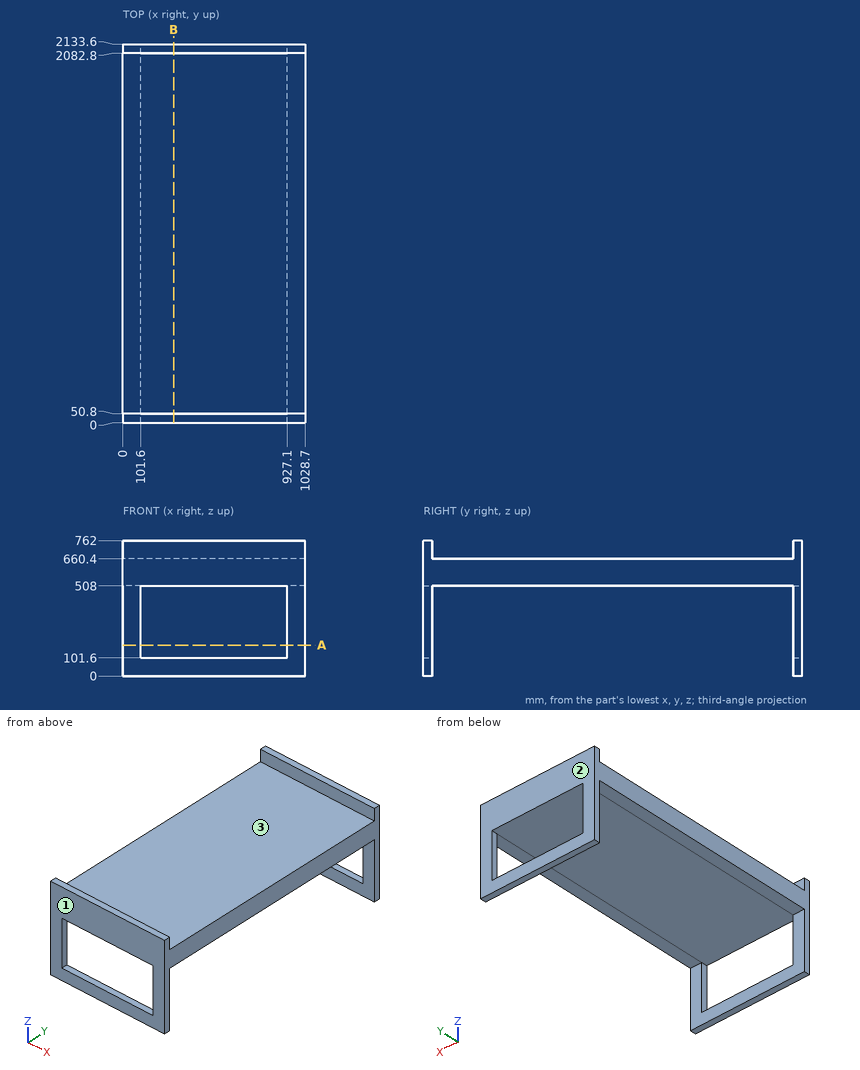
Could you check a few things on this drawing? It's one solid part, dimensions in mm from its lowest x, y, z. Coordinates: 2 decimals unless noted, no trailing zeros. Loops run counter-clockwise (first coordinate to the right, second up) from the corner with the lowest first, then second, coordinate; pieces in that order, holes last. Notation, with made-up numbers: (51, 35) - (81, 35) arc R22 ccw to (81, 59) - close; hole circle Ø11 at (34, -38). An arc over 180 degrees is marked (long way). Answer as a JSON object with one key per item and string values. Group by question number.
Item 1: If we section it at A-A (z = 174): List the corners of the cut face in (x, y) for me, plus the area to 3 significant figures.
Item 2: If we section it at B-B (x = 286): List the corners of the cut face in (y, z) for me, plus the area to 3 significant figures.
Item 3: If I drill on L1, parallel to Y at x = 59.5, z = 200; L2, parallel to Z at x = 387, y = 1585.5, over which ranges is the centre line in solid material (lowest first)? Write a range as from..to.
Item 4: For pin 1 (10 mm diameter, centred on x = 485.5, y = 619, fed in from -Z); pin 2 (1.5 mm diameter, centred on x = 588.5, y = 1878.5, fed in from +Z), each with a flat end and sliding along its axis, tell me the tip position at first contact or that it passes through.
Item 5: If we mould it in two halves opening along Y, with no side actions, what happens to the marked faces 1, 2 and 3? For each: released by +Y, released by -Y, zero draft, split by the parting line, or undercut.
Returned:
{
 "1": {"outline": "(0, 0) - (101.6, 0) - (101.6, 50.8) - (0, 50.8) - close; (0, 2082.8) - (101.6, 2082.8) - (101.6, 2133.6) - (0, 2133.6) - close; (927.1, 0) - (1028.7, 0) - (1028.7, 50.8) - (927.1, 50.8) - close; (927.1, 2082.8) - (1028.7, 2082.8) - (1028.7, 2133.6) - (927.1, 2133.6) - close", "area": "20,600 mm²"},
 "2": {"outline": "(0, 0) - (50.8, 0) - (50.8, 101.6) - (0, 101.6) - close; (0, 508) - (2133.6, 508) - (2133.6, 762) - (2082.8, 762) - (2082.8, 660.4) - (50.8, 660.4) - (50.8, 762) - (0, 762) - close; (2082.8, 0) - (2133.6, 0) - (2133.6, 101.6) - (2082.8, 101.6) - close", "area": "346,000 mm²"},
 "3": {"L1": "y = 0..50.8, 2082.8..2133.6", "L2": "z = 508..660.4"},
 "4": {"pin 1": "stops at z = 508", "pin 2": "stops at z = 660.4"},
 "5": {"face 1": "released by -Y", "face 2": "released by +Y", "face 3": "undercut"}
}
